Print and shaded views of the part. All mm, measured from the part's lowest x, y and z. A direction names the side the tool comes from. Give positions to 0.01 mm unless a question says otherwise; leave off trailing zeros. Write each loop counter-clockwise with the first axis right and the second up, starting at its lowest first coordinate (ties: lowest second). Pieces come first, ordered by that corner, then holes. Notation, with made-up numbers: M 3.25,16.25 L 29.25,16.25 A10 cw 29.25,34.25 Z; hole C 11.5,42 d9. An arc over 180 degrees is marked long. One line per question, with ' | ' between items. Start each with the question number.
1. Cut at B-B, the plane y = 61.5. Write the cut outline in (x, z), then the cut area to 3 significant figures.
2. Pull direction Y, two halves, no side cores. Call the marked faces 5, 6 and 7: released by +Y, released by -Y, zero draft, split by the parting line, or undercut.
3. Flat gauge pins, fed straight in: pin 1 (5 mm diameter, centred on x = 3.5, y = 3.5, fed in from +Z); pin 2 (3.5 mm diameter, centred on x = 61, z = 13.5, fed in from +Y); pin 3 (1 mm diameter, centred on x = 19, y = 38.5, fed in from +Z); pin 4 (6 mm diameter, centred on y = 58, z = 14, fed in from -X). Where does each tip first touch, or does it go through?
4. Cut at A-A, the plane z = 6. Write the cut outline in (x, y).
5. Which spindle directions (+Z, -Z, +X, -X, +Y, -Y) get a long thin tool onto all of the face, cutting with end or side? Do the marked faces 1, 2, 3 and 4. Say none if no direction does.
6. Cut at D-D, the plane x = 14. Write the cut outline in (y, z), then the cut area to 3 significant figures.
7. Wall check: L1, parallel to Y at x = 3.5, z = 2.4; L2, parallel to X at y = 15.5, z = 16.5. Give the ranges that are in metal, low to high.
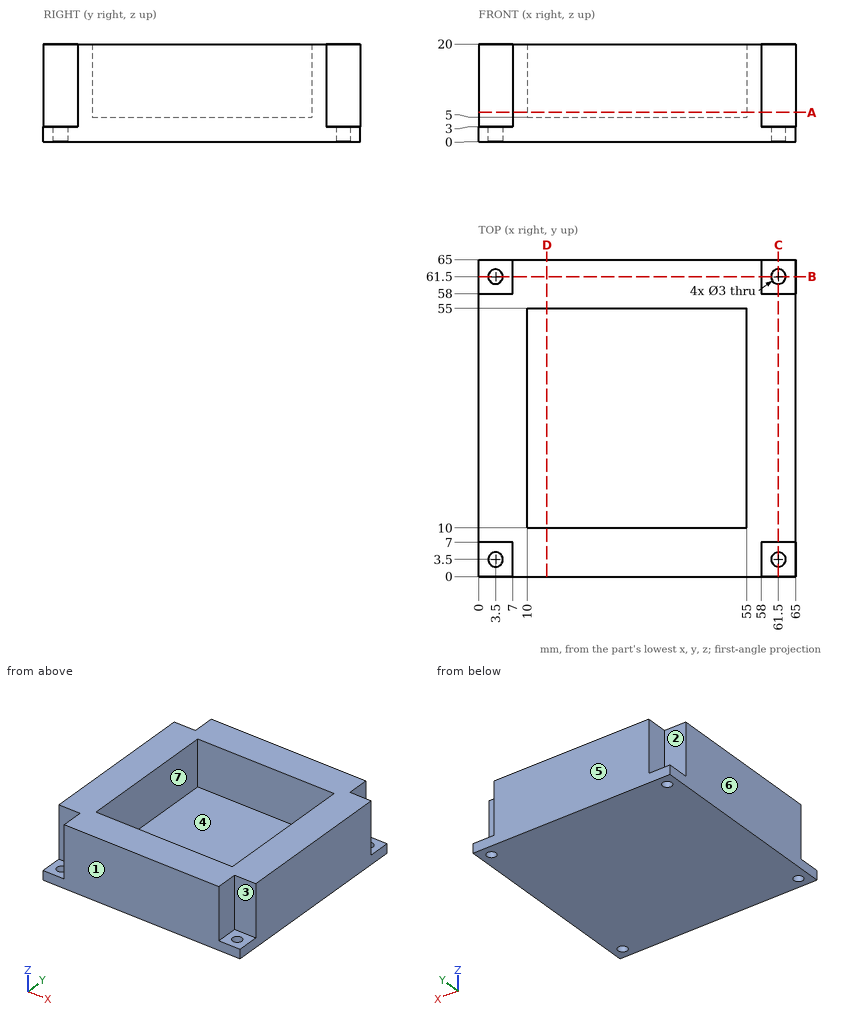
Here are the results:
1) outline: M 0,0 L 2,0 L 2,3 L 0,3 Z; M 5,0 L 60,0 L 60,3 L 58,3 L 58,20 L 7,20 L 7,3 L 5,3 Z; M 63,0 L 65,0 L 65,3 L 63,3 Z | area: 1,040 mm^2
2) face 5: released by +Y | face 6: zero draft | face 7: undercut
3) pin 1: z = 3 | pin 2: y = 58 | pin 3: z = 5 | pin 4: x = 0
4) outline: M 0,7 L 7,7 L 7,0 L 58,0 L 58,7 L 65,7 L 65,58 L 58,58 L 58,65 L 7,65 L 7,58 L 0,58 Z; hole M 10,10 L 55,10 L 55,55 L 10,55 Z
5) face 1: +Z, -Z, +X, -X, -Y | face 2: +Z, -X, +Y | face 3: +Z, +X, -Y | face 4: +Z
6) outline: M 0,0 L 65,0 L 65,20 L 55,20 L 55,5 L 10,5 L 10,20 L 0,20 Z | area: 625 mm^2
7) L1: 0 to 2, 5 to 60, 63 to 65 | L2: 0 to 10, 55 to 65
